Study the drawing (mm; zero at the part's minimum x, y, z) and answer. A direction names the side the tool comes from. Round coordinates to 2 decimals unless told otherwise and drop trailing zeros. Loops run counter-clockwise (first coordinate to the right, second up) from the corner with the lowest first, then second, coordinate; pieces in that order, holes last. Notation, with made-up numbers: (70.5, -25) - (115.5, -25) arc R19 ccw to (115.5, -11) - close; hole circle Ø7 at (88, 63.5). An arc over 180 degrees is marked (long way). Use CSV: the item, a comma, the result in double quotes. Start each with the question number.
1. Determine the mould class of the marked faces 6, 7 and 8 for opening direction X: +X half, -X half, draft (parallel to the pull), parting line (faces both ways), or undercut.
2. A tool of negligible diameter and unlimited length cuts with its end or side. For the marked faces 1, 2, 3, 4 and 5, from which of +Z, -Z, +X, -X, +Y, -Y can it reach the whole face along a straight path? Write none if from no direction.
3. Find section A-A (x = 14.5). State how many separate pieces and enclosed holes the cut face has.
4. Find section D-D (z = 1.75). Give the vertices of the cut face in (x, y), and give its area (3 significant figures).
5. Given pin 1 Ø6 at (y, z) = (38.5, 2.5) entering from +X; pin 2 Ø3 at (x, z) = (8, 5.5) entering from +Y; pin 3 Ø3 at (y, z) = (27, 4) entering from -X, each flat-ended and moving along its own axis, determine where each tip first touches the part or whether it passes through.
6. Find section B-B (x = 10.5). Give the vertices of the cut face in (y, z).
7. Consider line 1 along Y through (x, z) = (22, 6.25); line 2 along Z through (x, y) = (14.85, 47.25) (1 decimal); line 3 along X through (y, z) = (9, 3.75). Determine where each line is inside the solid, lowest interval first.
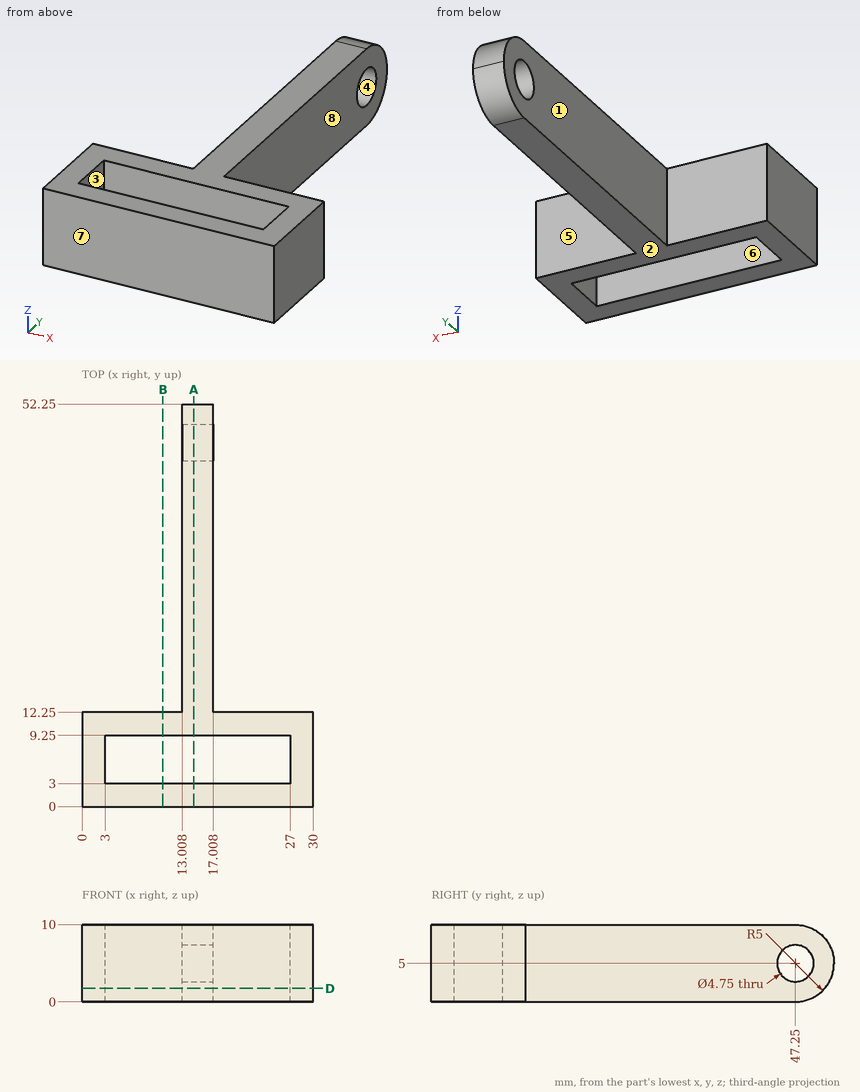
Filled sheet:
1,face 6,"undercut"
1,face 7,"draft"
1,face 8,"+X half"
2,face 1,"+Z, -Z, -X, +Y"
2,face 2,"-Z, +X, -X, +Y, -Y"
2,face 3,"+Z, -Z"
2,face 4,"+X, -X"
2,face 5,"+Z, -Z, +X, +Y"
3,separate pieces,"2"
3,enclosed holes,"1"
4,outline,"(0, 0) - (30, 0) - (30, 12.25) - (17.01, 12.25) - (17.01, 51.05) - (13.01, 51.05) - (13.01, 12.25) - (0, 12.25) - close; hole (3, 3) - (27, 3) - (27, 9.25) - (3, 9.25) - close"
4,area,"373 mm²"
5,pin 1,"stops at x = 17.01"
5,pin 2,"stops at y = 12.25"
5,pin 3,"stops at x = 13.01"
6,outline,"(0, 0) - (3, 0) - (3, 10) - (0, 10) - close; (9.25, 0) - (12.25, 0) - (12.25, 10) - (9.25, 10) - close"
7,line 1,"y = 0 to 3, 9.25 to 12.25"
7,line 2,"z = 0 to 2.6, 7.4 to 10"
7,line 3,"x = 0 to 3, 27 to 30"
